from build123d import *

# Parameters (mm, degrees)
RESSALTO_EXTRUS_O1_DEPTH                             = 4
FILETE1_R                                            = 4
CHANFRO1_SIZE                                        = 1
FURO_DE_DI_METRO_7_0_7_1_D                           = 7
ESCAREADO_PARA_PARAFUSO_COM_CABE_A_ESCAR_D           = 3.4
ESCAREADO_PARA_PARAFUSO_COM_CABE_A_ESCAR_CSINK_D     = 6.3
ESCAREADO_PARA_PARAFUSO_COM_CABE_A_ESCAR_CSINK_ANGLE = 90
BROCA_DE_ROSQUEAR_PARA_TARRAXA_DE_M21_D              = 1.6
BROCA_DE_ROSQUEAR_PARA_TARRAXA_DE_M21_DEPTH          = 8
BROCA_DE_ROSQUEAR_PARA_TARRAXA_DE_M21_TIP            = 0.480688495
FURO_DE_DI_METRO_9_0_9_3_D                           = 9
ESCAREADO_PARA_PARAFUSO_ALLEN_SEXTAVADO_D            = 3.4
ESCAREADO_PARA_PARAFUSO_ALLEN_SEXTAVADO_CSINK_D      = 6.72
ESCAREADO_PARA_PARAFUSO_ALLEN_SEXTAVADO_CSINK_ANGLE  = 90
ESCAREADO_PARA_PARAFUSO_COM_CABE_A_E_2_D             = 3.4
ESCAREADO_PARA_PARAFUSO_COM_CABE_A_E_2_DEPTH         = 4
ESCAREADO_PARA_PARAFUSO_COM_CABE_A_E_2_CSINK_D       = 6.3
ESCAREADO_PARA_PARAFUSO_COM_CABE_A_E_2_CSINK_ANGLE   = 90
ESCAREADO_PARA_PARAFUSO_COM_CABE_A_E_2_TIP           = 1.021463052
ESBO_O12_R                                           = 4.55
CORTE_EXTRUS_O1_DEPTH                                = 3
FURO_DE_DI_METRO_3_5_3_5_1_D                         = 3.5
ESBO_O36_R                                           = 12.5
CORTE_EXTRUS_O4_DEPTH                                = 2
ESCAREADO_PARA_PARAFUSO_ALLEN_SEXTAV_2_D             = 3.4
ESCAREADO_PARA_PARAFUSO_ALLEN_SEXTAV_2_CSINK_D       = 6.72
ESCAREADO_PARA_PARAFUSO_ALLEN_SEXTAV_2_CSINK_ANGLE   = 90
ESCAREADO_PARA_PARAFUSO_ALLEN_SEXTAV_2_O_D           = 3.4
ESCAREADO_PARA_PARAFUSO_ALLEN_SEXTAV_2_O_CSINK_D     = 6.72
ESCAREADO_PARA_PARAFUSO_ALLEN_SEXTAV_2_O_CSINK_ANGLE = 90


with BuildPart() as part:
    # Esboço1 → Ressalto-extrusão1 (new body)
    with BuildSketch(Plane.XY):
        Polygon((0, 0), (22, 0), (22, 80), (0, 75), align=None)
    extrude(amount=RESSALTO_EXTRUS_O1_DEPTH)

    # Filete1
    filete1_edges = [part.edges().sort_by_distance(p)[0] for p in [
        (0, 75, 2),
        (22, 80, 2),
    ]]
    fillet(filete1_edges, radius=FILETE1_R)

    # Chanfro1
    chanfro1_edges = [part.edges().sort_by_distance(p)[0] for p in [
        (10.113515586, 77.298526269, 0),
        (0, 35.903542878, 0),
        (0.873825208, 74.302487761, 0),
        (20.495402006, 78.115078729, 0),
        (22, 37.494451969, 0),
    ]]
    chamfer(chanfro1_edges, length=CHANFRO1_SIZE)

    # Furo de diâmetro Ø7.0 (7)1 (through all)
    with Locations(Plane(origin=(7.780869527, 38.393713373, 0), x_dir=(-1, 0, 0), z_dir=(0, 0, -1))):
        with Locations((0, 0)):
            Hole(FURO_DE_DI_METRO_7_0_7_1_D / 2)

    # Escareado para parafuso com cabe_a escar (through all)
    with Locations(Plane(origin=(18, 7, 0), x_dir=(-1, 0, 0), z_dir=(0, 0, -1))):
        with Locations((0, 0), (0, 7)):
            CounterSinkHole(ESCAREADO_PARA_PARAFUSO_COM_CABE_A_ESCAR_D / 2, ESCAREADO_PARA_PARAFUSO_COM_CABE_A_ESCAR_CSINK_D / 2, counter_sink_angle=ESCAREADO_PARA_PARAFUSO_COM_CABE_A_ESCAR_CSINK_ANGLE)

    # Broca de rosquear para tarraxa de M21
    with Locations(Plane(origin=(4, 0, 2), x_dir=(0, 0, -1), z_dir=(0, -1, 0))):
        with Locations((0, 0), (0, 8)):
            Hole(BROCA_DE_ROSQUEAR_PARA_TARRAXA_DE_M21_D / 2, depth=BROCA_DE_ROSQUEAR_PARA_TARRAXA_DE_M21_DEPTH)
            with Locations((0, 0, -(BROCA_DE_ROSQUEAR_PARA_TARRAXA_DE_M21_DEPTH + BROCA_DE_ROSQUEAR_PARA_TARRAXA_DE_M21_TIP / 2))):  # 118° drill point
                Cone(0, BROCA_DE_ROSQUEAR_PARA_TARRAXA_DE_M21_D / 2, BROCA_DE_ROSQUEAR_PARA_TARRAXA_DE_M21_TIP, mode=Mode.SUBTRACT)

    # Furo de diâmetro Ø9.0 (9)3 (through all)
    with Locations(Plane(origin=(7.780869527, 60.893713373, 0), x_dir=(-1, 0, 0), z_dir=(0, 0, -1))):
        with Locations((0, 0)):
            Hole(FURO_DE_DI_METRO_9_0_9_3_D / 2)

    # Escareado para parafuso Allen sextavado (through all)
    with Locations(Plane(origin=(14.368851738, 55.36573993, 0), x_dir=(-1, 0, 0), z_dir=(0, 0, -1))):
        with Locations((0, 0), (13.175964422, 11.055946886)):
            CounterSinkHole(ESCAREADO_PARA_PARAFUSO_ALLEN_SEXTAVADO_D / 2, ESCAREADO_PARA_PARAFUSO_ALLEN_SEXTAVADO_CSINK_D / 2, counter_sink_angle=ESCAREADO_PARA_PARAFUSO_ALLEN_SEXTAVADO_CSINK_ANGLE)

    # Escareado para parafuso com cabe_a e 2
    with Locations(Plane(origin=(18, 30, 0), x_dir=(-1, 0, 0), z_dir=(0, 0, -1))):
        with Locations((0, 0)):
            CounterSinkHole(ESCAREADO_PARA_PARAFUSO_COM_CABE_A_E_2_D / 2, ESCAREADO_PARA_PARAFUSO_COM_CABE_A_E_2_CSINK_D / 2, depth=ESCAREADO_PARA_PARAFUSO_COM_CABE_A_E_2_DEPTH, counter_sink_angle=ESCAREADO_PARA_PARAFUSO_COM_CABE_A_E_2_CSINK_ANGLE)
            with Locations((0, 0, -(ESCAREADO_PARA_PARAFUSO_COM_CABE_A_E_2_DEPTH + ESCAREADO_PARA_PARAFUSO_COM_CABE_A_E_2_TIP / 2))):  # 118° drill point
                Cone(0, ESCAREADO_PARA_PARAFUSO_COM_CABE_A_E_2_D / 2, ESCAREADO_PARA_PARAFUSO_COM_CABE_A_E_2_TIP, mode=Mode.SUBTRACT)

    # Esboço12 → Corte-extrusão1 (cut)
    with BuildSketch(Plane.XY.offset(4)):
        with Locations((7.780869527, 38.393713373)):
            Circle(ESBO_O12_R)
    extrude(amount=-CORTE_EXTRUS_O1_DEPTH, mode=Mode.SUBTRACT)

    # Furo de diâmetro Ø3.5 (3.5)1 (through all)
    with Locations(Plane(origin=(3, 14, 0), x_dir=(-1, 0, 0), z_dir=(0, 0, -1))):
        with Locations((0, 0)):
            Hole(FURO_DE_DI_METRO_3_5_3_5_1_D / 2)

    # Esboço36 → Corte-extrusão4 (cut)
    with BuildSketch(Plane.XY.offset(4)):
        with Locations((7.780869527, 60.893713373)):
            Circle(ESBO_O36_R)
    extrude(amount=-CORTE_EXTRUS_O4_DEPTH, mode=Mode.SUBTRACT)

    # Escareado para parafuso Allen sextav 2 (through all)
    with Locations(Plane(origin=(7.780869527, 26.893713373, 4), x_dir=(1, 0, 0), z_dir=(0, 0, 1))):
        with Locations((0, 0)):
            CounterSinkHole(ESCAREADO_PARA_PARAFUSO_ALLEN_SEXTAV_2_D / 2, ESCAREADO_PARA_PARAFUSO_ALLEN_SEXTAV_2_CSINK_D / 2, counter_sink_angle=ESCAREADO_PARA_PARAFUSO_ALLEN_SEXTAV_2_CSINK_ANGLE)

    # Escareado para parafuso Allen sextav 2 o (through all)
    with Locations(Plane(origin=(7.780869527, 68.893713373, 2), x_dir=(1, 0, 0), z_dir=(0, 0, 1))):
        with Locations((0, 0)):
            CounterSinkHole(ESCAREADO_PARA_PARAFUSO_ALLEN_SEXTAV_2_O_D / 2, ESCAREADO_PARA_PARAFUSO_ALLEN_SEXTAV_2_O_CSINK_D / 2, counter_sink_angle=ESCAREADO_PARA_PARAFUSO_ALLEN_SEXTAV_2_O_CSINK_ANGLE)


solid = part.part
Can you work these out from the model? Positions are in its coordinate system, mm. A direction names the side the tool comes from. Give positions to 0.01 mm unless a question says otherwise; leave off trailing zeros. One line per item, written item: value.
1) Please list where these lines run through material, in increasing order: line 1 (X direction, y = 2, z = 2); line 2 (Y direction, x = 2.75, z = 3.3); line 3 (Y direction, x = 18, z = 2.65).
Geometry check:
line 1: x = 0 to 3.2, 4.8 to 11.2, 12.8 to 22
line 2: y = 0 to 12.27, 15.73 to 49.45, 72.34 to 75.61
line 3: y = 0 to 5.3, 8.7 to 12.3, 15.7 to 28.3, 31.7 to 53.7, 68.09 to 78.99
2) Thinking about a two-plate mould opening in X: for faces 3 (the face through (7.325, 41.864, 0.507)), 4 (the face through (13, 40, 0)), 5 (the face through (0.897, 74.332, 2.521)), which applies, +X half, -X half, draft (parallel to the pull), parting line (faces both ways), or undercut?
Geometry check:
face 3: undercut
face 4: draft
face 5: -X half
3) I'm going to push flat-ended pins straight in: pin 1 (10.5 mm diameter, centred on x = 7.78, y = 38.39, fed in from +Z); pin 2 (3 mm diameter, centred on x = 1.19, y = 66.42, fed in from +Z); pin 3 (1.4 mm diameter, centred on x = 12, z = 2, fed in from +Y); pin 4 (1 mm diameter, centred on x = 4, z = 2, fed in from -Y). Where does each tip first touch, or does it pass through?
Geometry check:
pin 1: stops at z = 4
pin 2: passes through
pin 3: stops at y = 77.89
pin 4: stops at y = 8.18
4) On a 3-axis mill with a long thin cutter (end or side, diameter ignored), from which of +Z, -Z, +X, -X, +Y, -Y can I reach the whole of each face in a straight line? I mean faces 1 (the face through (0, 26, 2)), 2 (the face through (12, 58, 2)). Say none if no direction works.
Geometry check:
face 1: +Z, -Z, -X, +Y, -Y
face 2: +Z
